```python
from build123d import *

# Parameters (mm, degrees)
BOSS_EXTRUDE1_DEPTH = 10
M4_TAPPED_HOLE1_D   = 3.3
FILLET1_R           = 1


with BuildPart() as part:
    # Sketch1 → Boss-Extrude1 (new body)
    with BuildSketch(Plane(origin=(0, 0, 0), x_dir=(0, 0, -1), z_dir=(1, 0, 0))):
        with BuildLine():
            ThreePointArc((25, 57.609374237), (12.766583292, 61.488652214), (0, 62.8))
            ThreePointArc((0, 62.8), (-12.766583292, 61.488652214), (-25, 57.609374237))
            Line((-25, 57.609374237), (-25, 51.929182547))
            ThreePointArc((-25, 51.929182547), (-25.220795702, 51.145833095), (-25.818181818, 50.593097233))
            ThreePointArc((-25.818181818, 50.593097233), (-43.035646203, 37.069841595), (-53.859344034, 18.039153533))
            ThreePointArc((-53.859344034, 18.039153533), (-54.405495004, 17.298046479), (-55.281685866, 17.01553963))
            Line((-55.281685866, 17.01553963), (-59.5, 17.01553963))
            ThreePointArc((-59.5, 17.01553963), (-60.560660172, 16.576199802), (-61, 15.51553963))
            Line((-61, 15.51553963), (-61, 2.01553963))
            Line((-61, 2.01553963), (-50.76, 2.01553963))
            ThreePointArc((-50.76, 2.01553963), (0, 50.8), (50.76, 2.01553963))
            Line((50.76, 2.01553963), (61, 2.01553963))
            Line((61, 2.01553963), (61, 15.51553963))
            ThreePointArc((61, 15.51553963), (60.560660172, 16.576199802), (59.5, 17.01553963))
            Line((59.5, 17.01553963), (55.281685866, 17.01553963))
            ThreePointArc((55.281685866, 17.01553963), (54.405495004, 17.298046479), (53.859344034, 18.039153533))
            ThreePointArc((53.859344034, 18.039153533), (43.035646203, 37.069841595), (25.818181818, 50.593097233))
            ThreePointArc((25.818181818, 50.593097233), (25.220795702, 51.145833095), (25, 51.929182547))
            Line((25, 51.929182547), (25, 57.609374237))
        make_face()
    extrude(amount=BOSS_EXTRUDE1_DEPTH)

    # M4 Tapped Hole1 (through all)
    with Locations(Plane.XZ.offset(-2.01553963)):
        with Locations((5, -56), (5, 56)):
            Hole(M4_TAPPED_HOLE1_D / 2)

    # Fillet1
    fillet1_edges = [part.edges().sort_by_distance(p)[0] for p in [
        (5, 57.609374237, -25),
        (5, 57.609374237, 25),
    ]]
    fillet(fillet1_edges, radius=FILLET1_R)


solid = part.part
```
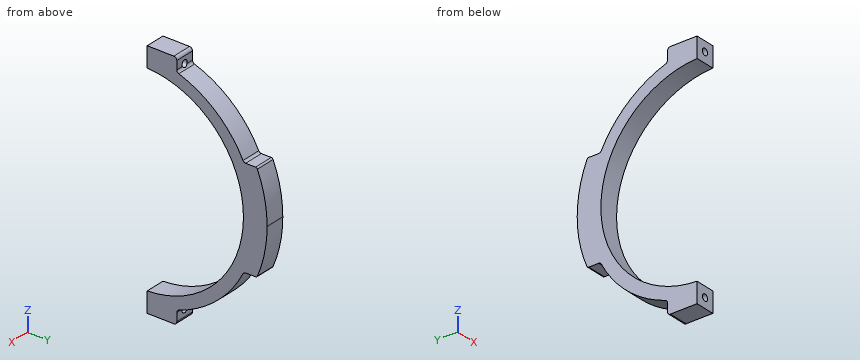
The listing builds one solid part. Answer for the finished solid, in the listing's coordinates (mm). Round coordinates to 2 decimals unless told otherwise and drop trailing zeros. Write each loop counter-clockwise with the first axis right and the second up, starting at its lowest first coordinate (ties: lowest second). Pieces come first, ordered by that corner, then holes. Notation, with made-up numbers: (-13, -3) -> (1, -3) arc R13 ccw to (1, 5) -> close; hole circle Ø9 at (76.5, -5). An arc over 180 degrees is marked (long way). Write item = value, one per line.
1) Given pin 1 (4 mm diameter, centred on x = 5, z = -56, fed in from +Y); pin 2 (2.5 mm diameter, centred on x = 4.5, y = 54, fed in from -Z); pin 3 (4 mm diameter, centred on x = 3.5, y = 54.5, fed in from +Z), each flat-ended and moving along its own axis, determine where each tip first touches the part or whether it passes through.
Check values:
pin_1 = 17.74
pin_2 = -25
pin_3 = 25
2) Section D-D on z = -18.5 is taken. Write down the section's boundary in (x, y), plus the area to 3 significant figures.
Check values:
outline = (0, 47.31) -> (10, 47.31) -> (10, 60.01) -> (0, 60.01) -> close
area = 127 mm²
3) Section C-C on y = 28 is taken. Write down the section's boundary in (x, z).
Check values:
outline = (0, -49.42) -> (10, -49.42) -> (10, -42.39) -> (0, -42.39) -> close; (0, 42.39) -> (10, 42.39) -> (10, 49.42) -> (0, 49.42) -> close
4) Section B-B on y = 44 is taken. Write down the section's boundary in (x, z).
Check values:
outline = (0, -35.92) -> (10, -35.92) -> (10, -25.39) -> (0, -25.39) -> close; (0, 25.39) -> (10, 25.39) -> (10, 35.92) -> (0, 35.92) -> close
5) Straight lines are drawn through the part: line 1 along Z through (x, y) = (5, 8); line 2 along X through (y, z) = (13.5, 56); line 3 along Z through (x, y) = (5, 9). For each, find the intervals that lie inside material, in ascending order. Write a range as [from, to].
Check values:
line_1 = [-61, -57.65], [-54.35, -50.17], [50.17, 54.35], [57.65, 61]
line_2 = [0, 3.35], [6.65, 10]
line_3 = [-61, -57.65], [-54.35, -50], [50, 54.35], [57.65, 61]
6) Section A-A on x = 5 is taken. Write down the section's boundary in (y, z), plus the area to 3 significant figures.
Check values:
outline = (2.02, -61) -> (15.52, -61) arc R1.5 ccw to (17.02, -59.5) -> (17.02, -57.65) -> (2.02, -57.65) -> close; (2.02, -54.35) -> (17.34, -54.35) arc R1.5 cw to (18.04, -53.86) arc R56.8 ccw to (50.59, -25.82) arc R1.5 cw to (51.93, -25) -> (56.95, -25) arc R1 ccw to (57.87, -24.39) arc R62.8 ccw to (57.87, 24.39) arc R1 ccw to (56.95, 25) -> (51.93, 25) arc R1.5 cw to (50.59, 25.82) arc R56.8 ccw to (18.04, 53.86) arc R1.5 cw to (17.34, 54.35) -> (2.02, 54.35) -> (2.02, 50.76) arc R50.8 cw to (2.02, -50.76) -> close; (2.02, 57.65) -> (17.02, 57.65) -> (17.02, 59.5) arc R1.5 ccw to (15.52, 61) -> (2.02, 61) -> close
area = 1,360 mm²
